Autodesk Inventor part; units mm, degrees
ref_plane "YZ Plane" through (0, 0, 0) normal (1, 0, 0) x (0, 1, 0)
ref_plane "XZ Plane" through (0, 0, 0) normal (0, 1, 0) x (-1, 0, 0)
ref_plane "XY Plane" through (0, 0, 0) normal (0, 0, 1) x (1, 0, 0)
sketch "Sketch1" plane through (0, 0, 0) normal (0, 1, 0) x (-1, 0, 0)
  line L0 (0, 0) -> (180, 0)
  line L1 (180, 0) -> (180, -32)
  line L2 (180, -32) -> (0, -32)
  line L3 (0, -32) -> (0, 0)
  line L4 (0, -32) -> (180, -32)
  line L5 (180, -32) -> (180, -29)
  line L6 (180, -29) -> (0, -29)
  line L7 (0, -29) -> (0, -32)
  line L8 (0, -32) -> (3, -32)
  line L9 (3, -32) -> (3, 0)
  line L10 (3, 0) -> (0, 0)
  line L11 (0, 0) -> (0, -32)
  line L12 (135.5, -29) -> (109.5, -29)
  line L13 (109.5, -29) -> (109.5, -13.5)
  line L14 (109.5, -13.5) -> (135.5, -13.5)
  line L15 (135.5, -13.5) -> (135.5, -29)
  line L16 (109.5, -29) -> (77.5, -29)
  line L17 (77.5, -29) -> (77.5, -11.5)
  line L18 (77.5, -11.5) -> (109.5, -11.5)
  line L19 (109.5, -11.5) -> (109.5, -29)
  line L20 (77.5, -29) -> (45.5, -29)
  line L21 (45.5, -29) -> (45.5, -9.5)
  line L22 (45.5, -9.5) -> (77.5, -9.5)
  line L23 (77.5, -9.5) -> (77.5, -29)
  line L24 (45.5, -29) -> (3, -29)
  line L25 (3, -29) -> (3, -6.25)
  line L26 (3, -6.25) -> (45.5, -6.25)
  line L27 (45.5, -6.25) -> (45.5, -29)
  point P0 (3, -29)
  point P1 (0, -29)
  dimension "d0" = 180
  dimension "d1" = 32
  dimension "d2" = 3
  dimension "d3" = 3
  dimension "d4" = 26
  dimension "d5" = 42.5
  dimension "d6" = 32
  dimension "d7" = 32
  dimension "d14" = 18.5
  dimension "d16" = 20.5
  dimension "d17" = 22.5
  dimension "d18" = 25.75
extrude "Extrusion1" add sketch "Sketch1" along normal blind 3 contours L0 L9 L6 L3 | L0 L1 L6 L15 L14 L19 L18 L23 L22 L27 L26 L9 | L6 L9 L2 L3 | L6 L1 L2 L9
properties part number "sledPlate" material "Polycarbonate, Smoke"
The model under review builds one solid part; all positions refer to its coordinate system, in mm. A direction names the side the tool comes from. Coordinates: 2 decimals unless noted, no trailing zeros. Write each loop counter-clockwise with the first axis right and the second up, starting at its lowest first coordinate (ties: lowest second). Pieces come first, ordered by that corner, then holes. Notation, with made-up numbers: (86.25, 25) - (113.25, 25) arc R13 ccw to (113.25, 44) - close; hole circle Ø9 at (-15, 6). An arc over 180 degrees is marked (long way). Answer as a JSON object with one key per item and string values. Group by question number.
1. Machinability: for faces 4 (the face through (-135.5, 1, -21)), 5 (the face through (-109, 3, -9)), which of the approach directions +Z, -Z, +X, -X, +Y, -Y give a long, thin tool a straight path to every point of the face, cutting with its end or side? Answer none if there is none.
2. Add section A-A (x = -125.5). Give the boundary of the cut face in (y, z).
3. Add section B-B (z = -23.5). Give the boundary of the cut face in (x, y).
4. Add section C-C (y = 1.1). Give the boundary of the cut face in (x, z), plus the area to 3 significant figures.
5. Mouldability with a two-part tool opening along Z and no side actions: class faces 1 (the face through (0, 1, -16)), 2 (the face through (-91, 1, -32)), 3 (the face through (-45.5, 1, -8)) as pulls with the +Z half, pulls with the -Z half, needs draft (parallel to the pull), parting line crosses it, or undercut.
6. To check wall thickness, follow probe 1 along Z at (x, y) = (-52, 2.5); probe 2 along X at (y, z) = (0.45, -9); probe 3 along Z at (x, y) = (-93, 0.85). State the ranges of each line that lie inside material, in increasing order.
Findings:
{
 "1": {"face 4": "+Y, -Y", "face 5": "+Z, -Z, +X, -X, +Y"},
 "2": {"outline": "(0, -32) - (3, -32) - (3, -29) - (0, -29) - close; (0, -13.5) - (3, -13.5) - (3, 0) - (0, 0) - close"},
 "3": {"outline": "(-180, 0) - (-135.5, 0) - (-135.5, 3) - (-180, 3) - close; (-3, 0) - (0, 0) - (0, 3) - (-3, 3) - close"},
 "4": {"outline": "(-180, -32) - (0, -32) - (0, 0) - (-180, 0) - close; hole (-135.5, -29) - (-3, -29) - (-3, -6.25) - (-45.5, -6.25) - (-45.5, -9.5) - (-77.5, -9.5) - (-77.5, -11.5) - (-109.5, -11.5) - (-109.5, -13.5) - (-135.5, -13.5) - close", "area": "3,210 mm²"},
 "5": {"face 1": "needs draft", "face 2": "pulls with the -Z half", "face 3": "undercut"},
 "6": {"probe 1": "-32 to -29, -9.5 to 0", "probe 2": "-180 to -45.5, -3 to 0", "probe 3": "-32 to -29, -11.5 to 0"}
}
